Verification items for this drawing (mm, ordinates from the low corner). Give positions to 0.01 mm unless a question says otherwise; leave off trailing zeros. Loops run counter-clockwise (first coordinate to the right, second up) from the corner with the lowest first, then second, coordinate; pieces in that order, holes last. Notation, with made-up numbers: (-12, 74) -> (-7, 74) arc R15 ccw to (-7, 98) -> close; hole circle Ø2 at (-34.75, 10.5). An arc over 180 degrees is marked (long way). Answer in a Markdown table with one row per item. Add a question column.
Q1. Material ranges on probe 1 along X at (y, z) = (1.1, 21); probe 2 along X at (y, z) = (1.9, 22.25); probe 3 along Z at (x, y) = (13, 3.5), recorded low to high.
Q2. Section check B-B on x = 20. Enter the section's corners in (y, z).
Q3. Section check A-A on z = 21. Enter the section's corners in (x, y), and give its area (3 significant figures).
Q4. Section check C-C on y = 2.05. Enter the section's corners in (x, z), and give its area (3 significant figures).
Q5. Release check for a two-part mould opening along Z. For the marked faces 1, 2 and 3 record: pulls with the +Z half, pulls with the -Z half, needs draft (parallel to the pull), parting line crosses it, or undercut.
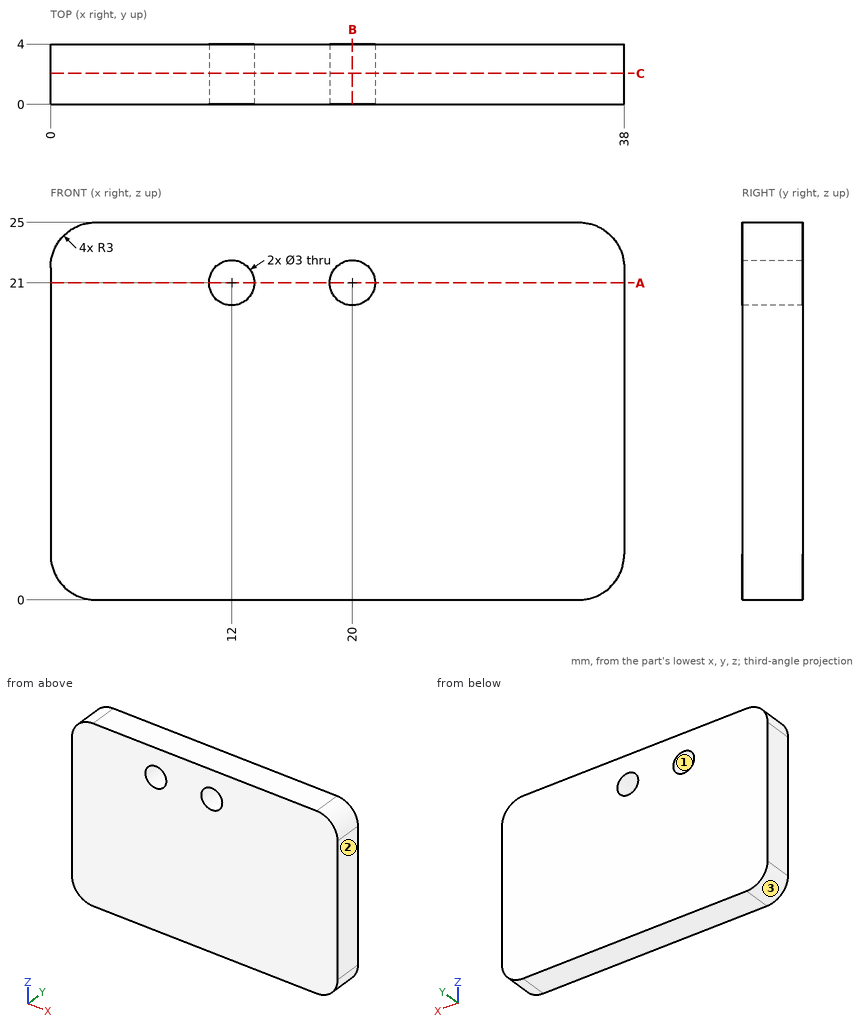
Taken from the geometry:
| question | item | result |
|---|---|---|
| 1 | probe 1 | x = 0 to 10.5, 13.5 to 18.5, 21.5 to 38 |
| 1 | probe 2 | x = 0.01 to 11.17, 12.83 to 19.17, 20.83 to 37.99 |
| 1 | probe 3 | z = 0 to 19.88, 22.12 to 25 |
| 2 | outline | (0, 0) -> (4, 0) -> (4, 19.5) -> (0, 19.5) -> close; (0, 22.5) -> (4, 22.5) -> (4, 25) -> (0, 25) -> close |
| 3 | outline | (0, 0) -> (10.5, 0) -> (10.5, 4) -> (0, 4) -> close; (13.5, 0) -> (18.5, 0) -> (18.5, 4) -> (13.5, 4) -> close; (21.5, 0) -> (38, 0) -> (38, 4) -> (21.5, 4) -> close |
| 3 | area | 128 mm² |
| 4 | outline | (0, 3) arc R3 ccw to (3, 0) -> (35, 0) arc R3 ccw to (38, 3) -> (38, 22) arc R3 ccw to (35, 25) -> (3, 25) arc R3 ccw to (0, 22) -> close; hole circle Ø3 at (12, 21); hole circle Ø3 at (20, 21) |
| 4 | area | 928 mm² |
| 5 | face 1 | undercut |
| 5 | face 2 | needs draft |
| 5 | face 3 | pulls with the -Z half |
